Can you work these out from the drawing? Everything is in mm from the part's minimum corner. Round coordinates to 2 decimals unless told otherwise and drop trailing zeros. Write each loop counter-clockwise with the first axis right and the second up, starting at its lowest first coordinate (ties: lowest second). Pieces come first, ordered by that corner, then holes. Notation, with made-up numbers: (57, 0.5) -> (77, 0.5) arc R19 cw to (77, 14.5) -> close; hole circle Ø11 at (18.25, 37.25). An arc over 180 degrees is marked (long way). Answer as CSV lines item,"result".
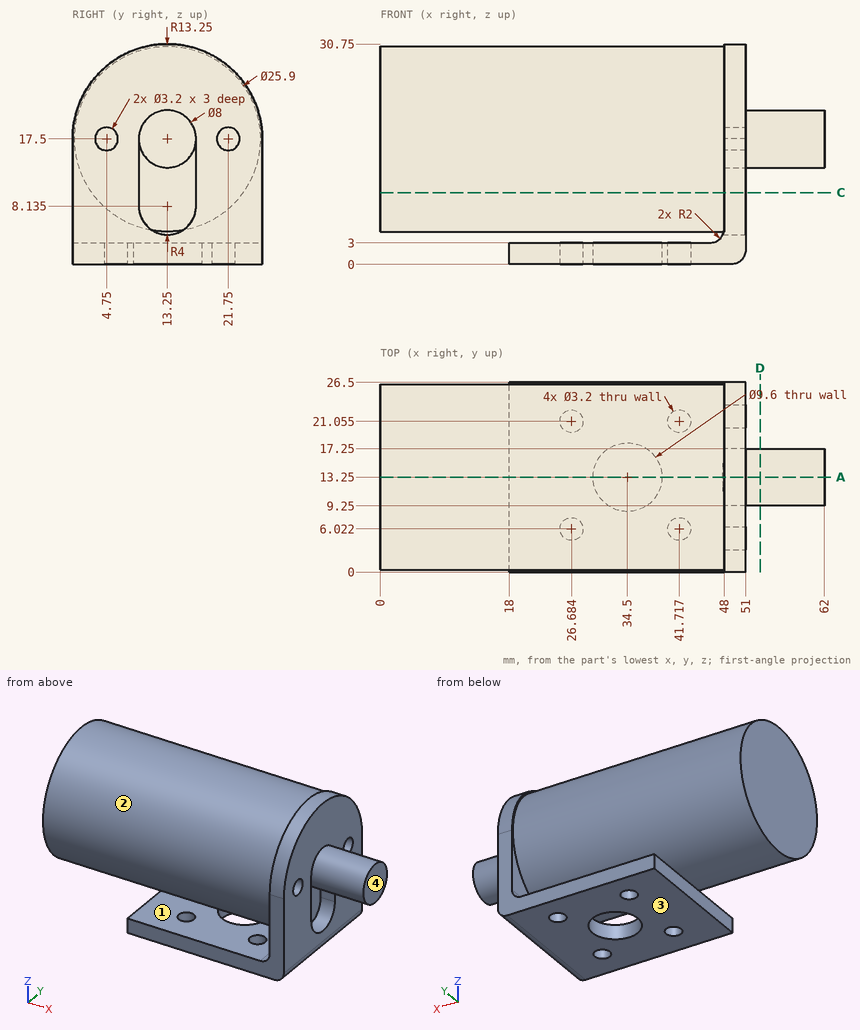
Item 1: I need wall thicknesses on L1, parallel to Y at x = 34.5, z = 0.85; L2, parallel to X at y = 19, z = 23; L3, parallel to X at y = 10, z = 8.5. Which ranges of each line are inside material? Lowest first, please.
Results found:
L1,"y = 0 to 8.45, 18.05 to 26.5"
L2,"x = 0 to 51"
L3,"x = 0 to 48"
Item 2: If we mould it in two halves opening along Z, with no side actions, what happens to the marked faces 1, 2, 3 and 4? For each: pulls with the +Z half, pulls with the -Z half, needs draft (parallel to the pull), parting line crosses it, or undercut.
Results found:
face 1,"undercut"
face 2,"undercut"
face 3,"pulls with the -Z half"
face 4,"needs draft"
Item 3: Suppose I cut it at C-C, the plane z = 10. List the corners of the cut face in (x, y) for me, then the cut area to 3 significant figures.
Results found:
outline,"(0, 2.69) -> (48, 2.69) -> (48, 0) -> (51, 0) -> (51, 9.25) -> (48, 9.25) -> (48, 17.25) -> (51, 17.25) -> (51, 26.5) -> (48, 26.5) -> (48, 23.81) -> (0, 23.81) -> close"
area,"1,070 mm²"
Item 4: Suppose I cut it at A-A, the plane y = 13.25. State how many separate pieces and enclosed holes the cut face has, then the cut area to 3 significant figures.
Results found:
separate pieces,"3"
enclosed holes,"0"
area,"1,460 mm²"
Item 5: Will these pins go through, and if not, where does the flat tip stop? pin 1 (1 mm diameter, centred on y = 3, z = 24.5, fed in from +X); pin 2 (1 mm diameter, centred on y = 5, z = 17.5, fed in from +X); pin 3 (1.5 mm diameter, centred on y = 9.5, z = 1.5, fed in from -X).
Results found:
pin 1,"stops at x = 51"
pin 2,"stops at x = 48"
pin 3,"stops at x = 18"
Item 6: Suppose I cut it at D-D, the plane x = 53. List the corners of the cut face in (y, z) for me.
Results found:
outline,"circle Ø8 at (13.25, 17.5)"
